Can you work these out from the model? Positions are in its coordinate system, mm. Face numbers are marked on the shaded views. A direction names the side the tool comes from. Give positions to 0.01 mm unless a question says otherwise; leave off trailing zeros. Order: outer loops, then holes, each group sorted by start corner. A loop starts at its lowest first (then second) coordinate and runs counter-clockwise, first axis right, second up. Notation, with made-up numbers: (-3, 62) -> (4, 62) arc R33 ccw to (4, 95) -> close; hole circle Ø10 at (8.25, -36.75). An arc over 180 degrees is marked (long way). Answer as CSV lines item,"result".
Autodesk Inventor part; units mm, degrees
ref_plane "YZ Plane" through (0, 0, 0) normal (1, 0, 0) x (0, 1, 0)
ref_plane "XZ Plane" through (0, 0, 0) normal (0, 1, 0) x (-1, 0, 0)
ref_plane "XY Plane" through (0, 0, 0) normal (0, 0, 1) x (1, 0, 0)
sketch "スケッチ1" plane through (0, 0, 0) normal (0, 0, 1) x (1, 0, 0)
  circle A0 centre (0, 0) radius 10
  dimension "d0" = 20
extrude "押し出し1" add sketch "スケッチ1" along normal blind 5
sketch "スケッチ2" plane through (0, 0, 5) normal (0, 0, 1) x (1, 0, 0)
  circle A0 centre (0, 0) radius 10
  circle A1 centre (0, 0) radius 11
  circle A2 centre (0, 0) radius 10
  dimension "d3" = 22
extrude "押し出し2" add sketch "スケッチ2" against normal blind 1
sketch "スケッチ3" plane through (0, 0, 0) normal (0, 0, -1) x (-1, 0, 0)
  point P0 (0, 0)
  point P1 (2, 0)
  dimension "d6" = 2
hole "穴1" at (-2, 0, 0) direction (0, 0, 1) diameter 8 end through all
sketch "スケッチ4" plane through (0, 0, 0) normal (0, 0, -1) x (-1, 0, 0)
  circle A0 centre (2, 0) radius 4
  line L0 (0.5, 3.7081) -> (3.5, 3.7081)
  line L1 (3.5, 3.7081) -> (3.5, 5.1081)
  line L2 (3.5, 5.1081) -> (0.5, 5.1081)
  line L3 (0.5, 5.1081) -> (0.5, 3.7081)
  circle A1 centre (2, 5.1081) radius 1.5
  point P0 (0, 0)
  point P1 (0.5, 5.1081)
  dimension "d14" = 3
  dimension "d15" = 1.4
extrude "押し出し3" cut sketch "スケッチ4" against normal through all contours L0 A1 A0 | A0 A1 L1 | L3 A1 A0 | A0 A1 L0 | A1 L0 A0 | A0 A1 L2 | L2 A1 picked at (3.1128, 3.733) picked at (0.8872, 3.733) picked at (2.0995, 3.8017)
properties part number "偏心軸板" material "アルミニウム 6061"
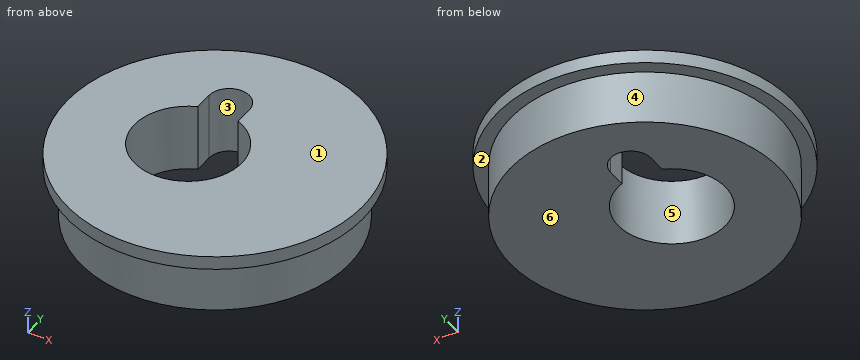
Item 1: Imagine slicing it at C-C, the plane z = 4.65. Please give me the cut outline in (x, y), then the cut area to 3 significant figures.
Numbers:
outline,"circle Ø22 at (0, 0); hole (-3.5, 3.71) arc R4 ccw (long way) to (-0.5, 3.71) -> (-0.5, 5.11) arc R1.5 ccw to (-3.5, 5.11) -> close"
area,"323 mm²"
Item 2: Imagine slicing it at B-B, the plane x = -4.75. Please give me the cut outline in (y, z), then the cut area to 3 significant figures.
Numbers:
outline,"(-9.92, 4) -> (-8.8, 4) -> (-8.8, 0) -> (-2.9, 0) -> (-2.9, 5) -> (-9.92, 5) -> close; (2.9, 0) -> (8.8, 0) -> (8.8, 4) -> (9.92, 4) -> (9.92, 5) -> (2.9, 5) -> close"
area,"61.2 mm²"
Item 3: For pin 1 (7 mm diameter, centred on x = -2, y = 0, fed in from +Z); pin 2 (1 mm diameter, centred on x = 6, z = 3, fed in from -Y); pin 3 (1 mm diameter, centred on y = 5, z = 1, fed in from -X), each with a flat end and sliding along its axis, tell me the tip position at first contact or that it passes through.
Numbers:
pin 1,"passes through"
pin 2,"stops at y = -8.35"
pin 3,"stops at x = -8.93"
Item 4: Please list where these lines run through material, in increasing order: line 1 along Z through (x, y) = (10, -3.5); line 2 along Y through (x, z) = (-1.5, 4.35); line 3 along X through (y, z) = (2.75, 3.65).
Numbers:
line 1,"z = 4 to 5"
line 2,"y = -10.9 to -3.97, 6.52 to 10.9"
line 3,"x = -9.61 to -4.9, 0.9 to 9.61"
Item 5: Imagine slicing it at A-A, the plane y = 0. Please give me the cut outline in (x, z).
Numbers:
outline,"(-11, 4) -> (-10, 4) -> (-10, 0) -> (-6, 0) -> (-6, 5) -> (-11, 5) -> close; (2, 0) -> (10, 0) -> (10, 4) -> (11, 4) -> (11, 5) -> (2, 5) -> close"
Item 6: We'd pull the mould along Y, two halves only. Please class the marked faces 3, 4, 5 and 6: released by +Y, released by -Y, zero draft, split by the parting line, or undercut.
Numbers:
face 3,"undercut"
face 4,"split by the parting line"
face 5,"undercut"
face 6,"zero draft"
Item 7: Imagine slicing it at D-D, the plane z = 1.75. Please give me the cut outline in (x, y), then the cut area to 3 significant figures.
Numbers:
outline,"circle Ø20 at (0, 0); hole (-3.5, 3.71) arc R4 ccw (long way) to (-0.5, 3.71) -> (-0.5, 5.11) arc R1.5 ccw to (-3.5, 5.11) -> close"
area,"257 mm²"
Item 8: For the marked faces 1 and 2, which set-ups out of +Z, -Z, +X, -X, +Y, -Y let a thin tool reach every point of the face, with its end or its side?
Numbers:
face 1,"+Z, +X, -X, +Y, -Y"
face 2,"-Z"
